Can you work these out from the model? Positions are in its coordinate system, mm. Face numbers are marked on the shaded views. A direction names the side the tool comes from. Give positions to 0.01 mm unless a question says otherwise; leave off trailing zeros. Order: outer loops, then holes, each group sorted by start corner. A loop starts at its lowest first (then second) coordinate and runs counter-clockwise, first axis right, second up. Notation, with made-up numbers: M 65.5,14.5 L 119.5,14.5 A31 ccw 119.5,39.5 Z; hole C 31.5,-35.5 d8. An arc over 180 degrees is marked long. Use one line per item in the form item = value. Start each with the question number.
1. For the marked faces 5, 6 and 7, which set-ups out of +Z, -Z, +X, -X, +Y, -Y let a thin tool reach every point of the face, with its end or its side?
2. I want a section at C-C, the plane z = 98. List the corners of the cut face in (x, y) for me (3 decimals).
3. I want a section at B-B, the plane y = 21. List the corners of the cut face in (x, z) for me, and give its area (3 significant figures).
4. I need wall thicknesses on L1, parallel to X at y = 52, z = 145; L2, parallel to X at y = 57.5, z = 99.5; L3, parallel to Z at x = -34, y = 25.5. Which ranges of each line are inside material? Lowest first, please.
5. We'd pull the mould along Z, two halves only. Please class the marked faces 1, 2, 3 and 4: +Z half, -Z half, draft (parallel to the pull), parting line (faces both ways), or undercut.
6. Will this pin go through, and if not, where does the flat tip stop? P1, Ø14.5, axis at x = -35, z = 138.5, coming from the -Y side.
7. I want a section at A-A, the plane x = 2. List the corners of the cut face in (y, z) for me (1 decimal), and give its area (3 significant figures).
```python
from build123d import *

# Parameters (mm, degrees)
SKETCH1_W           = 419.1
SKETCH1_H           = 333.375
BOSS_EXTRUDE1_DEPTH = 60.325
SKETCH2_W           = 139.7
SKETCH2_H           = 50.8
CUT_EXTRUDE1_DEPTH  = 61.325
CHAMFER1_SIZE       = 50.8
CHAMFER1_SIZE2      = 13.611818976
FILLET1_R           = 12.7
SKETCH3_W           = 139.7
SKETCH3_H           = 56.403006085
CUT_EXTRUDE2_DEPTH  = 12.7
SKETCH4_W           = 139.7
SKETCH4_H           = 56.128435861
CUT_EXTRUDE3_DEPTH  = 12.7


with BuildPart() as part:
    # Sketch1 → Boss-Extrude1 (new body)
    with BuildSketch(Plane(origin=(0, 0, 0), x_dir=(1, 0, 0), z_dir=(0, 1, 0))):
        Rectangle(SKETCH1_W, SKETCH1_H)
    extrude(amount=BOSS_EXTRUDE1_DEPTH)

    # Sketch2 → Cut-Extrude1 (cut, through all)
    with BuildSketch(Plane(origin=(0, 60.325, 0), x_dir=(1, 0, 0), z_dir=(0, 1, 0))):
        with Locations((0, -115.8875)):
            Rectangle(SKETCH2_W, SKETCH2_H)
        Polygon((-69.85, -166.6875), (-69.85, -157.1625), (-32.169017961, -166.6875), align=None)
        Polygon((32.169017961, -166.6875), (69.85, -166.6875), (69.85, -157.1625), align=None)
    extrude(amount=-CUT_EXTRUDE1_DEPTH, mode=Mode.SUBTRACT)

    # Chamfer1
    chamfer1_edges = [part.edges().sort_by_distance(p)[0] for p in [
        (69.85, 30.1625, 141.2875),
        (-69.85, 30.1625, 141.2875),
    ]]
    chamfer1_side = [part.faces().sort_by_distance(p)[0] for p in [
        (0, 30.1625, 141.2875),
    ]]
    chamfer(chamfer1_edges, length=CHAMFER1_SIZE, length2=CHAMFER1_SIZE2, reference=chamfer1_side[0])

    # Fillet1
    fillet1_edges = [part.edges().sort_by_distance(p)[0] for p in [
        (69.85, 30.1625, 90.4875),
        (-69.85, 30.1625, 90.4875),
        (-32.169017961, 30.1625, 166.6875),
        (32.169017961, 30.1625, 166.6875),
        (69.85, 30.1625, 127.675681024),
        (-19.05, 30.1625, 141.2875),
        (19.05, 30.1625, 141.2875),
        (-69.85, 30.1625, 127.675681024),
    ]]
    fillet(fillet1_edges, radius=FILLET1_R)

    # Sketch3 → Cut-Extrude2 (cut)
    with BuildSketch(Plane(origin=(0, 60.325, 0), x_dir=(1, 0, 0), z_dir=(0, 1, 0))):
        with Locations((0, -138.485996957)):
            Rectangle(SKETCH3_W, SKETCH3_H)
    extrude(amount=-CUT_EXTRUDE2_DEPTH, mode=Mode.SUBTRACT)

    # Sketch4 → Cut-Extrude3 (cut)
    with BuildSketch(Plane.XZ):
        with Locations((0, 138.623282069)):
            Rectangle(SKETCH4_W, SKETCH4_H)
    extrude(amount=-CUT_EXTRUDE3_DEPTH, mode=Mode.SUBTRACT)


solid = part.part
```
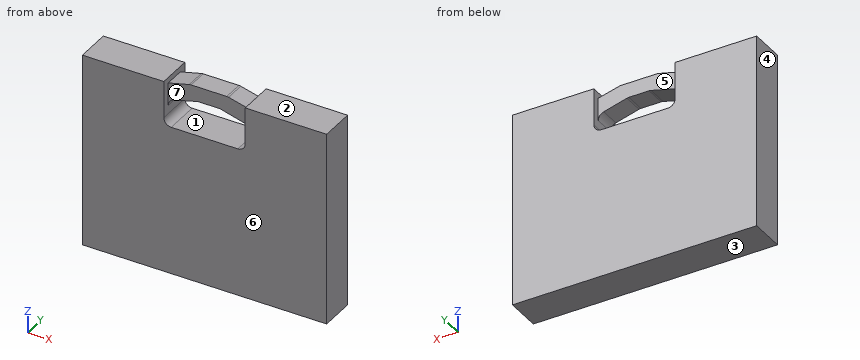
Check result:
q1.face_5 = +Z, +Y
q1.face_6 = +Z, -Z, +X, -X, -Y
q1.face_7 = +Z, -Y
q2.outline = M -209.55,0 L -68.742,0 L -68.742,60.325 L -209.55,60.325 Z; M 68.742,0 L 209.55,0 L 209.55,60.325 L 68.742,60.325 Z
q3.outline = M -209.55,-166.69 L 209.55,-166.69 L 209.55,166.69 L 69.85,166.69 L 69.85,157.16 L 33.7,166.3 A12.7 ccw 30.59,166.69 L -30.59,166.69 A12.7 ccw -33.7,166.3 L -69.85,157.16 L -69.85,166.69 L -209.55,166.69 Z; hole M -69.85,103.19 A12.7 ccw -57.15,90.49 L 57.15,90.49 A12.7 ccw 69.85,103.19 L 69.85,117.93 A12.7 ccw 60.44,130.2 L 20.67,140.85 A12.7 ccw 17.38,141.29 L -17.38,141.29 A12.7 ccw -20.67,140.85 L -60.44,130.2 A12.7 ccw -69.85,117.93 Z
q3.area = 133,000 mm2
q4.L1 = -209.55 to -69.85, 69.85 to 209.55
q4.L2 = -209.55 to -69.3, 69.3 to 209.55
q4.L3 = -166.69 to 90.49, 137.28 to 166.22
q5.face_1 = undercut
q5.face_2 = +Z half
q5.face_3 = -Z half
q5.face_4 = draft
q6.P1 = 12.7
q7.outline = M 0,-166.7 L 60.3,-166.7 L 60.3,90.5 L 0,90.5 Z; M 12.7,141.3 L 47.6,141.3 L 47.6,166.7 L 12.7,166.7 Z
q7.area = 16,400 mm2
